Solid Edge part; units mm, degrees
sketch "Sketch1" plane through (0, 0, 0) normal (0, 0, 1) x (1, 0, 0)
  line L0 (-6.5, -6.5) -> (6.5, -6.5)
  line L1 (6.5, -6.5) -> (6.5, 6.5)
  line L2 (6.5, 6.5) -> (-6.5, 6.5)
  line L3 (-6.5, 6.5) -> (-6.5, -6.5)
extrude "Protrusion1" add sketch "Sketch1" along normal blind 3
sketch "Sketch2" plane through (0, 0, 0) normal (0, 0, 1) x (1, 0, 0)
  line L0 (10.5, -6.5) -> (6.5, -6.5)
  line L1 (6.5, -6.5) -> (6.5, 6.5)
  line L2 (6.5, 6.5) -> (10.5, 6.5)
  line L3 (10.5, 6.5) -> (10.5, -6.5)
  line L4 (-6.5, -6.5) -> (-10.5, -6.5)
  line L5 (-10.5, -6.5) -> (-10.5, 6.5)
  line L6 (-10.5, 6.5) -> (-6.5, 6.5)
  line L7 (-6.5, 6.5) -> (-6.5, -6.5)
extrude "ExtrudedProtrusion_2" add sketch "Sketch2" along normal blind 14
sketch "Sketch3" plane through (10.5, 0, 7) normal (1, 0, 0) x (0, 1, 0)
  circle A0 centre (0, 1.5) radius 1.5
extrude "ExtrudedCutout_1" cut sketch "Sketch3" against normal blind 39
Could you check a few things on this model? Use its own coordinates, in mm. A direction names the side the tool comes from. Round coordinates to 2 decimals unless told otherwise and drop trailing zeros. Write each loop counter-clockwise with the first axis right and the second up, starting at its lowest first coordinate (ties: lowest second). Pieces come first, ordered by that corner, then holes. Notation, with made-up numbers: (-28, 54) -> (14, 54) arc R31 cw to (14, 90) -> close; hole circle Ø11 at (21.5, 54.5). An arc over 180 degrees is marked (long way). Use a Markdown table: item, result.
1. Please list where these lines run through material, in increasing order: probe 1 along X at (y, z) = (0.5, 6.25); probe 2 along Z at (x, y) = (8.65, 0); probe 3 along Z at (x, y) = (-6, 0.5).
Answer key:
| item | result |
|---|---|
| probe 1 | x = -10.5 to -6.5, 6.5 to 10.5 |
| probe 2 | z = 0 to 7, 10 to 14 |
| probe 3 | z = 0 to 3 |
2. If we section it at C-C (z = 4): List the corners of the cut face in (x, y) for me.
Answer key:
| item | result |
|---|---|
| outline | (-10.5, -6.5) -> (-6.5, -6.5) -> (-6.5, 6.5) -> (-10.5, 6.5) -> close; (6.5, -6.5) -> (10.5, -6.5) -> (10.5, 6.5) -> (6.5, 6.5) -> close |
3. If we section it at D-D (x = 7.25): List the corners of the cut face in (y, z) for me.
Answer key:
| item | result |
|---|---|
| outline | (-6.5, 0) -> (6.5, 0) -> (6.5, 14) -> (-6.5, 14) -> close; hole circle Ø3 at (0, 8.5) |
4. If we section it at A-A (z = 8.5): List the corners of the cut face in (x, y) for me.
Answer key:
| item | result |
|---|---|
| outline | (-10.5, -6.5) -> (-6.5, -6.5) -> (-6.5, -1.5) -> (-10.5, -1.5) -> close; (-10.5, 1.5) -> (-6.5, 1.5) -> (-6.5, 6.5) -> (-10.5, 6.5) -> close; (6.5, -6.5) -> (10.5, -6.5) -> (10.5, -1.5) -> (6.5, -1.5) -> close; (6.5, 1.5) -> (10.5, 1.5) -> (10.5, 6.5) -> (6.5, 6.5) -> close |
5. If we section it at B-B (y = 0): List the corners of the cut face in (x, z) for me, then the cut area to 3 significant figures.
Answer key:
| item | result |
|---|---|
| outline | (-10.5, 0) -> (10.5, 0) -> (10.5, 7) -> (6.5, 7) -> (6.5, 3) -> (-6.5, 3) -> (-6.5, 7) -> (-10.5, 7) -> close; (-10.5, 10) -> (-6.5, 10) -> (-6.5, 14) -> (-10.5, 14) -> close; (6.5, 10) -> (10.5, 10) -> (10.5, 14) -> (6.5, 14) -> close |
| area | 127 mm^2 |
6. We'd pull the mould along Z, two halves only. Please class faces 1 (the face through (-6.5, 2, 8)), 2 (the face through (-8, 0, 14)), 3 (the face through (-8, 0, 7)): +Z half, -Z half, draft (parallel to the pull), parting line (faces both ways), or undercut.
Answer key:
| item | result |
|---|---|
| face 1 | draft |
| face 2 | +Z half |
| face 3 | undercut |
7. Which directions (+Z, -Z, +X, -X, +Y, -Y) give clear straight access to the entire face, cutting with the end or side of a thin tool? Please do faces 4 (the face through (0, 0, 3)), 5 (the face through (0, 0, 0)).
Answer key:
| item | result |
|---|---|
| face 4 | +Z, +Y, -Y |
| face 5 | -Z, +X, -X, +Y, -Y |
8. For pin 1 Ø2.5 at (y, z) = (0, 8.5) entering from +X; pin 2 Ø6.5 at (x, y) = (2, 0.5) entering from +Z, each with a flat end and sliding along its axis, tell me the tip position at first contact or that it passes through.
Answer key:
| item | result |
|---|---|
| pin 1 | passes through |
| pin 2 | stops at z = 3 |
